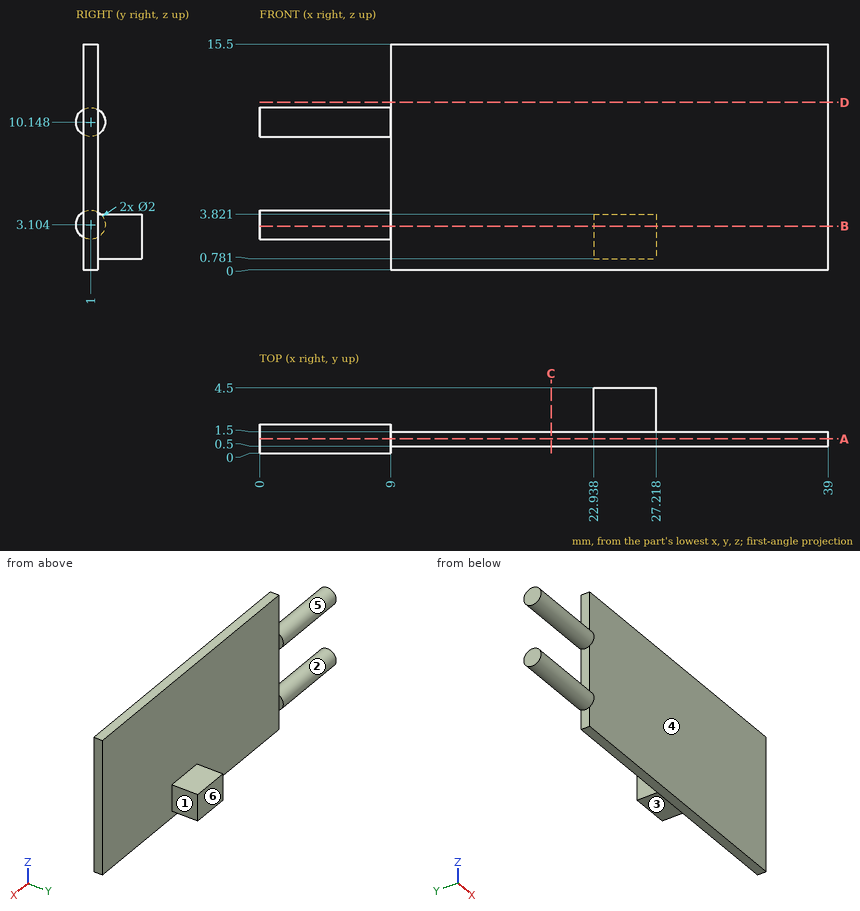
Job drawing, mm, ordinate dimensions from the low corner. One solid piece. A direction names the side the tool comes from. Coordinates: 2 decimals unless noted, no trailing zeros. Order: outer loops, then holes, each group sorted by start corner. A loop starts at its lowest first (then second) coordinate and runs counter-clockwise, first axis right, second up. Notation, with made-up numbers: M -28.75,-31.75 L 23.25,-31.75 A16 ccw 23.25,-3.75 Z; hole C 81.25,4 d5. An arc over 180 degrees is marked long. Answer as CSV lines item,"result".
(1) Band-saw the part on D-D, the plane z = 11.5. List the corners of the cut face in (x, y).
Geometry says:
outline,"M 9,0.5 L 39,0.5 L 39,1.5 L 9,1.5 Z"
(2) Flat gauge pins, fed straight in: pin 1 (1.5 mm diameter, centred on x = 25.5, y = 2.5, fed in from +Z); pin 2 (8 mm diameter, centred on x = 30.5, z = 9, fed in from +Y); pin 3 (0.8 mm diameter, centred on y = 1, z = 13, fed in from -X); pin 4 (2.5 mm diameter, centred on y = 2.5, z = 2, fed in from -X). Where does each tip first touch, or does it go through?
Geometry says:
pin 1,"stops at z = 3.82"
pin 2,"stops at y = 1.5"
pin 3,"stops at x = 9"
pin 4,"stops at x = 0"
(3) Band-saw the part on B-B, the plane z = 3. List the corners of the cut face in (x, y) (1 decimal).
Geometry says:
outline,"M 0,0 L 9,0 L 9,0.5 L 39,0.5 L 39,1.5 L 27.2,1.5 L 27.2,4.5 L 22.9,4.5 L 22.9,1.5 L 9,1.5 L 9,2 L 0,2 Z"
(4) Wall check: line 1 along Y through (x, z) = (35, 9.5); line 2 along X through (y, z) = (0.3, 10.5); line 3 along X through (y, z) = (2.15, 3.75). Give the ranges that are in metal, low to high.
Geometry says:
line 1,"y = 0.5 to 1.5"
line 2,"x = 0 to 9"
line 3,"x = 22.94 to 27.22"
(5) Pull direction Z, two halves, no side cores. Call the marked faces 1, 2 and 3: +Z half, -Z half, draft (parallel to the pull), parting line (faces both ways), or undercut.
Geometry says:
face 1,"draft"
face 2,"undercut"
face 3,"-Z half"
(6) 3-axis set-ups, long thin cutter, end or side, ignore diameter. For the marked faces 4, 5 and 6: which of +Z, -Z, +X, -X, +Y, -Y reach the whole face in a straight line?
Geometry says:
face 4,"+Z, -Z, +X, -Y"
face 5,"-X"
face 6,"+Z, -Z, +X, -X, +Y"
(7) Band-saw the part on A-A, the plane y = 1. List the corners of the cut face in (x, z), then the cut area to 3 significant figures.
Geometry says:
outline,"M 0,2.1 L 9,2.1 L 9,0 L 39,0 L 39,15.5 L 9,15.5 L 9,11.15 L 0,11.15 L 0,9.15 L 9,9.15 L 9,4.1 L 0,4.1 Z"
area,"501 mm2"
(8) Band-saw the part on C-C, the plane x = 20. List the corners of the cut face in (y, z), then the cut area to 3 significant figures.
Geometry says:
outline,"M 0.5,0 L 1.5,0 L 1.5,15.5 L 0.5,15.5 Z"
area,"15.5 mm2"
